Design review of the part built by this model. Coordinates are the model's own, in mm. Give positions to 0.01 mm unless a question says otherwise; leave off trailing zeros. Write each loop counter-clockwise with the first axis right and the second up, starting at its lowest first coordinate (ties: lowest second). Pieces come first, ordered by that corner, then holes. Notation, with made-up numbers: (-29, 29.5) - (-10, 29.5) arc R10 ccw to (-10, 37.5) - close; hole circle Ø10 at (45.5, 35.5). An arc over 180 degrees is marked (long way). Use a Markdown table: item, result. Add a question column.
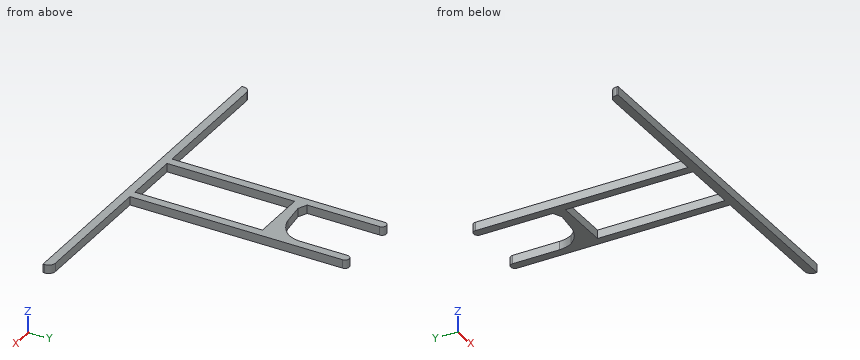
```python
from build123d import *

# Parameters (mm, degrees)
F0_W     = 3.175
F0_H     = 47.625
F1_DEPTH = 3.175


with BuildPart() as f1:
    # F0 (on Top) → F1 (new body)
    with BuildSketch(Plane.XY):
        with BuildLine():
            Line((0, 31.75), (0, 0))
            Line((0, 0), (3.175, 0))
            Line((3.175, 0), (24.003, 0))
            Line((24.003, 0), (27.178, 0))
            Line((27.178, 0), (27.178, 31.75))
            ThreePointArc((27.178, 31.75), (25.5905, 33.3375), (24.003, 31.75))
            Line((24.003, 31.75), (24.003, 14.16871))
            Line((24.003, 14.16871), (24.003, 11.557))
            Line((24.003, 11.557), (24.003, 5.207))
            Line((24.003, 5.207), (24.003, 3.175))
            Line((24.003, 3.175), (6.477, 3.175))
            Line((6.477, 3.175), (3.175, 3.175))
            Line((3.175, 3.175), (3.175, 4.699))
            Line((3.175, 4.699), (3.175, 31.75))
            ThreePointArc((3.175, 31.75), (1.5875, 33.3375), (0, 31.75))
        make_face()
        with Locations((1.5875, -23.8125)):
            Rectangle(F0_W, F0_H)
        Polygon((3.175, -47.625), (0, -47.625), (0, -50.8), (27.178, -50.8), (27.178, -47.625), (24.003, -47.625), align=None)
        with BuildLine():
            Line((0, -50.8), (0, -47.625))
            Line((0, -47.625), (-48.26, -47.625))
            ThreePointArc((-48.26, -47.625), (-50.056051, -48.368949), (-50.8, -50.165))
            Line((-50.8, -50.165), (-50.8, -50.8))
            Line((-50.8, -50.8), (0, -50.8))
        make_face()
        with Locations((25.5905, -23.8125)):
            Rectangle(F0_W, F0_H)
        Polygon((6.477, 3.175), (3.175, 4.699), (3.175, 3.175), align=None)
        with BuildLine():
            Line((27.178, -47.625), (27.178, -50.8))
            Line((27.178, -50.8), (77.978, -50.8))
            Line((77.978, -50.8), (77.978, -50.165))
            ThreePointArc((77.978, -50.165), (77.234051, -48.368949), (75.438, -47.625))
            Line((75.438, -47.625), (27.178, -47.625))
        make_face()
        Polygon((14.541382, 4.110001), (6.477, 3.175), (24.003, 3.175), (24.003, 5.207), align=None)
        with BuildLine():
            ThreePointArc((22.702671, 9.255895), (19.129717, 5.877759), (14.541382, 4.110001))
            Line((14.541382, 4.110001), (24.003, 5.207))
            Line((24.003, 5.207), (24.003, 11.557))
            ThreePointArc((24.003, 11.557), (23.412861, 10.372528), (22.702671, 9.255895))
        make_face()
        with BuildLine():
            ThreePointArc((24.003, 14.16871), (23.633619, 11.637984), (22.702671, 9.255895))
            ThreePointArc((22.702671, 9.255895), (23.412861, 10.372528), (24.003, 11.557))
            Line((24.003, 11.557), (24.003, 14.16871))
        make_face()
    extrude(amount=F1_DEPTH)


solid = f1.part
```
(1) Add section C-C (x = -34). State the section outline as (y, z) points (3 decimals), and give its area (3 significant figures).
(2) Add section B-B (y = -22). State the section outline as (x, z) points (3 decimals).
(3) For line 1 along X through (y, z) = (-42.5, 1.5) (3 decimals); line 2 along Y through (x, z) = (-8.5, 2.55) (3 decimals); line 3 along X through (y, z) = (1.5, 0.2), list the stretches that pass through material, from the lowest coordinate up.
(4) Insertion check: pin 1 (1 mm diameter, centred on y = 21.5, z = 1.5, fed in from +X); pin 2 (10 mm diameter, centred on x = 2.5, y = -5, fed in from -Z); pin 3 (1 mm diameter, centred on y = -18, z = 1, fed in from -X); pin 4 (1.5 mm diameter, centred on x = 46, z = 0.5, fed in from +Y) (3 decimals). Each pin has a flat end and moves straight along its axis. Give the tip position at first contact, or say it passes through.
Answers follow:
| question | item | result |
|---|---|---|
| 1 | outline | (-50.8, 0) - (-47.625, 0) - (-47.625, 3.175) - (-50.8, 3.175) - close |
| 1 | area | 10.1 mm^2 |
| 2 | outline | (0, 0) - (3.175, 0) - (3.175, 3.175) - (0, 3.175) - close; (24.003, 0) - (27.178, 0) - (27.178, 3.175) - (24.003, 3.175) - close |
| 3 | line 1 | 0 to 3.175, 24.003 to 27.178 |
| 3 | line 2 | -50.8 to -47.625 |
| 3 | line 3 | 0 to 27.18 |
| 4 | pin 1 | x = 27.18 |
| 4 | pin 2 | z = 0 |
| 4 | pin 3 | x = 0 |
| 4 | pin 4 | y = -47.625 |
